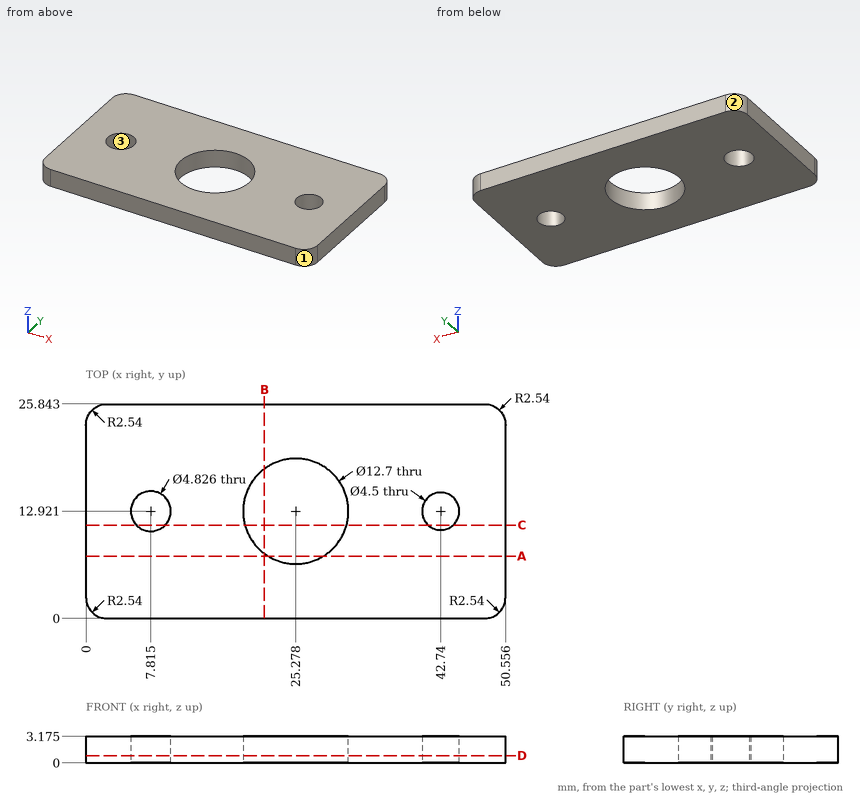
Study the drawing (mm; zero at the part's minimum x, y, z) and answer. Round coordinates to 2 decimals unless told otherwise and drop trailing zeros. Write each loop counter-clockwise with the first axis right and the second up, starting at its lowest first coordinate (ties: lowest second). Pieces come first, ordered by that corner, then holes. Notation, with made-up numbers: (85.25, 68) - (141.25, 68) arc R26 cw to (141.25, 87) - close; hole circle Ø10 at (35, -8). An arc over 180 degrees is marked (long way). Return JSON: item names as keys, results as strings. Group by question number.
Q1. The mould has two halves that part along X. Classify the marked faces 1, 2 and 3: released by +X, released by -X, zero draft, split by the parting line, or undercut.
Q2. The part is cut by section D-D on z = 0.85. Count the separate pieces of the cut face and the enclosed holes in it, then the cut area to 3 significant figures.
Q3. The part is cut by section B-B on x = 21.5. Write down the section's boundary in (y, z) (1 decimal).
Q4. Find the intervals of material crossed by L1, parallel to Y at x = 6.5, z = 2.7 (1 decimal); L2, parallel to X at y = 18.5, z = 1.95 (1 decimal); L3, parallel to X at y = 8, z = 2.85 (1 decimal), in increasing order.
Q5. The part is cut by section C-C on y = 11.25. Write down the section's boundary in (x, z) (1 decimal), then the cut area to 3 significant figures.
Q6. The part is cut by section A-A on y = 7.5. Write down the section's boundary in (x, z) (1 decimal).
Solved:
{
 "1": {"face 1": "released by +X", "face 2": "released by -X", "face 3": "undercut"},
 "2": {"separate pieces": "1", "enclosed holes": "3", "area": "1,140 mm²"},
 "3": {"outline": "(0, 0) - (7.8, 0) - (7.8, 3.2) - (0, 3.2) - close; (18, 0) - (25.8, 0) - (25.8, 3.2) - (18, 3.2) - close"},
 "4": {"L1": "0 to 10.9, 14.9 to 25.8", "L2": "0 to 22.2, 28.3 to 50.6", "L3": "0 to 21.3, 29.3 to 50.6"},
 "5": {"outline": "(0, 0) - (6.1, 0) - (6.1, 3.2) - (0, 3.2) - close; (9.6, 0) - (19.2, 0) - (19.2, 3.2) - (9.6, 3.2) - close; (31.4, 0) - (41.2, 0) - (41.2, 3.2) - (31.4, 3.2) - close; (44.2, 0) - (50.6, 0) - (50.6, 3.2) - (44.2, 3.2) - close", "area": "101 mm²"},
 "6": {"outline": "(0, 0) - (22, 0) - (22, 3.2) - (0, 3.2) - close; (28.6, 0) - (50.6, 0) - (50.6, 3.2) - (28.6, 3.2) - close"}
}
